from build123d import *

# Parameters (mm, degrees)
SKETCH1_R           = 2
BOSS_EXTRUDE1_DEPTH = 11.6
SKETCH2_R           = 4
BOSS_EXTRUDE2_DEPTH = 0.3
SKETCH3_R           = 8
BOSS_EXTRUDE3_DEPTH = 1
SKETCH4_R           = 1.5
CUT_EXTRUDE1_DEPTH  = 8.5
CUT_EXTRUDE2_DEPTH  = 17.419805115
CHAMFER1_SIZE       = 0.1


with BuildPart() as part:
    # Sketch1 → Boss-Extrude1 (new body)
    with BuildSketch(Plane(origin=(0, 0, 0), x_dir=(1, 0, 0), z_dir=(0, 1, 0))):
        with Locations(Location((0, 0, 0), (0, 0, 270))):
            Circle(SKETCH1_R)
    extrude(amount=BOSS_EXTRUDE1_DEPTH)

    # Sketch2 → Boss-Extrude2 (add)
    with BuildSketch(Plane(origin=(0, 11.6, 0), x_dir=(1, 0, 0), z_dir=(0, 1, 0))):
        with Locations(Location((0, 0, 0), (0, 0, 270))):
            Circle(SKETCH2_R)
    extrude(amount=BOSS_EXTRUDE2_DEPTH)

    # Sketch3 → Boss-Extrude3 (add)
    with BuildSketch(Plane(origin=(0, 11.9, 0), x_dir=(1, 0, 0), z_dir=(0, 1, 0))):
        with Locations(Location((0, 0, 0), (0, 0, 270))):
            Circle(SKETCH3_R)
    extrude(amount=BOSS_EXTRUDE3_DEPTH)

    # Sketch4 → Cut-Extrude1 (cut)
    with BuildSketch(Plane.XZ):
        with Locations(Location((0, 0, 0), (0, 0, 270))):
            Circle(SKETCH4_R)
    extrude(amount=-CUT_EXTRUDE1_DEPTH, mode=Mode.SUBTRACT)

    # Sketch5 → Cut-Extrude2 (cut, through all)
    with BuildSketch(Plane.XZ.offset(-11.9)):
        with BuildLine():
            ThreePointArc((1.5, -6), (1.060660172, -4.939339828), (0, -4.5))
            Line((0, -4.5), (0, -7.5))
            ThreePointArc((0, -7.5), (1.060660172, -7.060660172), (1.5, -6))
        make_face()
        with BuildLine():
            Line((0, -7.5), (0, -4.5))
            ThreePointArc((0, -4.5), (-1.5, -6), (0, -7.5))
        make_face()
    extrude(amount=-CUT_EXTRUDE2_DEPTH, mode=Mode.SUBTRACT)

    # Chamfer1
    chamfer1_edges = [part.edges().sort_by_distance(p)[0] for p in [
        (0, 12.9, -8),
        (0, 0, -2),
        (0, 11.6, -2),
        (0, 11.9, -8),
    ]]
    chamfer(chamfer1_edges, length=CHAMFER1_SIZE)


solid = part.part
Read the model definition and answer for the solid it produces. Units are mm, in the model's axes. A direction names the side the tool comes from. Give positions to 0.01 mm unless a question says otherwise; leave off trailing zeros. Loops run counter-clockwise (first coordinate to the right, second up) from the corner with the lowest first, then second, coordinate; pieces in that order, holes last. Notation, with made-up numbers: M 85.25,40 L 124.25,40 A18 cw 124.25,46 Z; hole C 79,31.25 d4. An arc over 180 degrees is marked long. Write each question's results on one line, items separated by ' | '.
1. Straight lines are drawn through the part: line 1 (X direction, y = 4.5, z = 0); line 2 (Y direction, x = -0.5, z = 3.25); line 3 (Y direction, x = 4.25, z = -3.5). For each, find the intervals that lie inside material, in ascending order. Write a range as [from, to].
Values:
line 1: x = [-2, -1.5], [1.5, 2] | line 2: y = [11.6, 12.9] | line 3: y = [11.9, 12.9]
2. Section C-C on y = 9.5 is taken. Give the vertices of the cut face in (x, z).
Values:
outline: C 0,0 d4
3. The mould has two halves that part along X. Classify faces 3 (the face through (0, 8.5, 0)), 4 (the face through (-7.81, 12.39, -1.73)), 5 (the face through (-2, 11.6, 2)): pulls with the +X half, pulls with the -X half, needs draft (parallel to the pull), parting line crosses it, or undercut.
Values:
face 3: undercut | face 4: parting line crosses it | face 5: needs draft
4. Section B-B on y = 4.75 is taken. Give the vertices of the cut face in (x, z), plus the area to 3 significant figures.
Values:
outline: C 0,0 d4; hole C 0,0 d3 | area: 5.50 mm^2
5. Given pin 1 (6 mm diameter, centred on x = -3.5, z = -4.5, fed in from -Y); pin 2 (5 mm diameter, centred on y = 7, z = 0, fed in from -X); pin 3 (1 mm diameter, centred on x = 3.5, z = 3, fed in from -Y), each flat-ended and moving along its own axis, determine where each tip first touches the part or whether it passes through.
Values:
pin 1: stops at y = 11.6 | pin 2: stops at x = -2 | pin 3: stops at y = 11.9
6. A tool of negligible diameter and unlimited length cuts with its end or side. For faces 1 (the face through (-2, 6, 0)), 2 (the face through (0, 12.9, 0)), from which of +Z, -Z, +X, -X, +Y, -Y can it reach the whole face along a straight path? Write none if from no direction.
Values:
face 1: -Y | face 2: +Z, -Z, +X, -X, +Y
7. Section A-A on z = 0 is taken. Give the vertices of the cut face in (x, y).
Values:
outline: M -8,12 L -7.9,11.9 L -4,11.9 L -4,11.6 L -2.1,11.6 L -2,11.5 L -2,0.1 L -1.9,0 L -1.5,0 L -1.5,8.5 L 1.5,8.5 L 1.5,0 L 1.9,0 L 2,0.1 L 2,11.5 L 2.1,11.6 L 4,11.6 L 4,11.9 L 7.9,11.9 L 8,12 L 8,12.8 L 7.9,12.9 L -7.9,12.9 L -8,12.8 Z
